Source: CAD feature listing. Evaluate the final solid. Frame: model axes, mm. A direction names the side the tool comes from. Coordinates: 2 decimals unless noted, no trailing zeros. Write each loop counter-clockwise with the first axis right and the second up, starting at its lowest first coordinate (ties: lowest second). Pieces come first, ordered by that corner, then holes. Notation, with made-up numbers: (23.5, 73) - (44.5, 73) arc R22 ccw to (44.5, 98) - close; hole circle Ø3 at (-10, 60.5). An arc over 180 degrees is marked (long way). One line per question, with ' | ' between items.
from build123d import *

# Parameters (mm, degrees)
SKETCH1_W            = 35
SKETCH1_H            = 15
BASE_FLANGE1_DEPTH   = 2
EDGE_FLANGE1_START   = -17.5
EDGE_FLANGE1_DEPTH   = 35
EDGE_FLANGE1_2_DEPTH = 35
EDGE_FLANGE2_START   = -17.5
EDGE_FLANGE2_DEPTH   = 35
EDGE_FLANGE2_2_DEPTH = 35
SKETCH8_W            = 25
SKETCH8_H            = 56.677305051
CUT_EXTRUDE1_DEPTH   = 10
BOSS_EXTRUDE1_DEPTH  = 2
BOSS_EXTRUDE2_DEPTH  = 2
M3_CLEARANCE_HOLE1_D = 3.6
M3_CLEARANCE_HOLE2_D = 3.6
M3_CLEARANCE_HOLE3_D = 3.6
M3_CLEARANCE_HOLE4_D = 3.6


# Read off the part's stored shape, not the designer's step: Edge-Flange1, Edge-Flange2
# Sheet-metal steps are written as plain solids
with BuildPart() as part:
    # Sketch1 → Base-Flange1 (new body)
    with BuildSketch(Plane.XY):
        Rectangle(SKETCH1_W, SKETCH1_H)
    extrude(amount=-BASE_FLANGE1_DEPTH)

    # Edge-Flange1 outline → Edge-Flange1 (cut)
    with BuildSketch(Plane.YZ.offset(EDGE_FLANGE1_START)):
        with BuildLine():
            ThreePointArc((-2.964101615, -2), (-3.999377795, -1.863703305), (-4.964101615, -1.464101615))
            Line((-4.964101615, -1.464101615), (-7.5, 0))
            Line((-7.5, 0), (-7.5, -2))
            Line((-7.5, -2), (-2.964101615, -2))
        make_face()
    extrude(amount=EDGE_FLANGE1_DEPTH, mode=Mode.SUBTRACT)

    # Edge-Flange1 2 outline → Edge-Flange1 2 (add)
    with BuildSketch(Plane.YZ.offset(EDGE_FLANGE1_START)):
        with BuildLine():
            Line((-65.708341645, 33.606601718), (-7.5, 0))
            Line((-7.5, 0), (-2.964101615, 0))
            ThreePointArc((-2.964101615, 0), (-3.481739705, 0.068148347), (-3.964101615, 0.267949192))
            Line((-3.964101615, 0.267949192), (-64.708341645, 35.338652525))
            Line((-64.708341645, 35.338652525), (-65.708341645, 33.606601718))
        make_face()
    extrude(amount=EDGE_FLANGE1_2_DEPTH)

    # Edge-Flange2 outline → Edge-Flange2 (cut)
    with BuildSketch(Plane.YZ.offset(EDGE_FLANGE2_START)):
        with BuildLine():
            ThreePointArc((-62.708341645, 31.87455091), (-64.17244326, 33.338652525), (-64.708341645, 35.338652525))
            Line((-64.708341645, 35.338652525), (-65.708341645, 33.606601718))
            Line((-65.708341645, 33.606601718), (-62.708341645, 31.87455091))
        make_face()
    extrude(amount=EDGE_FLANGE2_DEPTH, mode=Mode.SUBTRACT)

    # Edge-Flange2 2 outline → Edge-Flange2 2 (add)
    with BuildSketch(Plane.YZ.offset(EDGE_FLANGE2_START)):
        with BuildLine():
            Line((-64.708341645, 48.029251449), (-64.708341645, 35.338652525))
            Line((-64.708341645, 35.338652525), (-61.708341645, 33.606601718))
            ThreePointArc((-61.708341645, 33.606601718), (-62.440392453, 34.338652525), (-62.708341645, 35.338652525))
            Line((-62.708341645, 35.338652525), (-62.708341645, 48.029251449))
            Line((-62.708341645, 48.029251449), (-64.708341645, 48.029251449))
        make_face()
    extrude(amount=EDGE_FLANGE2_2_DEPTH)

    # Sketch8 → Cut-Extrude1 (cut)
    with BuildSketch(Plane(origin=(0, -0.875, -1.515544457), x_dir=(1, 0, 0), z_dir=(0, 0.499999999999995, 0.8660254037844416))):
        with Locations((0, -36.905639824)):
            Rectangle(SKETCH8_W, SKETCH8_H)
    extrude(amount=-CUT_EXTRUDE1_DEPTH, mode=Mode.SUBTRACT)

    # Sketch9 → Boss-Extrude1 (add)
    with BuildSketch(Plane(origin=(0, -0.875, -1.515544457), x_dir=(1, 0, 0), z_dir=(0, 0.499999999999995, 0.8660254037844416))):
        Polygon((8.83956854, -68.632858088), (7.246458748, -62.687291403), (15.857586038, -60.3799468), (15.081128903, -57.482169321), (6.470001613, -59.789513924), (1.919269462, -42.805950327), (15.365688048, -39.202993325), (14.946719777, -36.202993325), (1.14120391, -39.902170153), (-2.665166674, -25.696601742), (16.123001013, -20.662327383), (15.50761088, -17.662327383), (-3.456389996, -22.743716103), (-8.33426209, -4.539249615), (-11.232039569, -5.31570675), (-8.495960417, -15.52689316), (-17.05592393, -17.82052847), (-16.279466794, -20.718305949), (-7.708625485, -18.465267128), (-3.822054178, -32.970148713), (-15.793222539, -36.177813607), (-15.040127716, -39.177813607), (-3.021606391, -35.957460524), (1.177204702, -51.627636855), (-15.406874361, -56.071327447), (-14.947395895, -59.071327447), (1.957983923, -54.541544577), (5.941791061, -69.409315224), align=None)
    extrude(amount=-BOSS_EXTRUDE1_DEPTH)

    # Sketch10 → Boss-Extrude2 (add)
    with BuildSketch(Plane(origin=(0, -0.875, -1.515544457), x_dir=(1, 0, 0), z_dir=(0, 0.499999999999995, 0.8660254037844416))):
        Polygon((-3.456389996, -22.743716103), (12.5, -8.566987298), (10.507436864, -6.324289782), (-5.448953132, -20.501018587), align=None)
        Polygon((-2.665166674, -25.696601742), (12.5, -36.858589914), (14.278322137, -34.442483464), (-0.886844536, -23.280495293), align=None)
        Polygon((-3.822054178, -32.970148713), (-12.5, -19.724787915), (-15.00938766, -21.368860167), (-6.331441838, -34.614220965), align=None)
        Polygon((-12.5, -55.29243281), (-3.021606391, -35.957460524), (-5.715342898, -34.636936526), (-15.193736507, -53.971908812), align=None)
        Polygon((6.470001613, -59.789513924), (12.5, -39.970852124), (15.37009296, -40.844102603), (9.340094573, -60.662764404), align=None)
        Polygon((-12.5, -58.415549694), (4.825776546, -65.244292349), (3.725723751, -68.035328689), (-13.600052794, -61.206586033), align=None)
    extrude(amount=-BOSS_EXTRUDE2_DEPTH)

    # M3 Clearance Hole1 (through all)
    with Locations(Plane(origin=(-15.830402425, -63.569767603, -87), x_dir=(-1, 0, 0), z_dir=(0, 0, -1))):
        with Locations((-25.330402425, 65.569767603), (-6.330402425, 65.739876607)):
            Hole(M3_CLEARANCE_HOLE1_D / 2)

    # M3 Clearance Hole2 (through all)
    with Locations(Plane(origin=(15.830402425, -63.569767603, 0), x_dir=(1, 0, 0), z_dir=(0, 0, 1))):
        with Locations((-25.330402425, 65.569767603), (-6.330402425, 65.739876607)):
            Hole(M3_CLEARANCE_HOLE2_D / 2)

    # M3 Clearance Hole3 (through all)
    with Locations(Plane(origin=(15.830402425, -62.708341645, 22.375161803), x_dir=(-1, 0, 0), z_dir=(0, 1, 0))):
        with Locations((25.330402425, 19.654089646), (6.330402425, 19.654089646)):
            Hole(M3_CLEARANCE_HOLE3_D / 2)

    # M3 Clearance Hole4 (through all)
    with Locations(Plane(origin=(-15.830402425, -62.708341645, -109.375161803), x_dir=(1, 0, 0), z_dir=(0, 1, 0))):
        with Locations((25.330402425, -151.404413252), (6.330402425, -151.404413252)):
            Hole(M3_CLEARANCE_HOLE4_D / 2)


solid = part.part
Item 1: Pin query (flat end, axial travel): pin 1 Ø11.5 at (x, y) = (-1.5, 3.5) entering from +Z; pin 2 Ø1 at (x, y) = (6, -7) entering from -Z; pin 3 Ø14 at (x, z) = (-6, 43.5) entering from +Y. Return the tip coordinate at first contact, or that it passes through.
Check sheet entries:
pin 1: z = 0 | pin 2: z = -0.58 | pin 3: y = -62.71
Item 2: Ray query, line 1 along Y through (x, z) = (-7, 44.5); line 2 along Z through (x, y) = (9.5, -63.45); line 3 along Z through (x, y) = (9, -64). Return the intervals inside material, ascending. Write a range as [from, to].
Check sheet entries:
line 1: [-64.71, -62.71] | line 2: [32.43, 40.23], [43.83, 48.03] | line 3: [33.07, 40.3], [43.76, 48.03]
Item 3: Mould query, pull axis X, two halves, no side actions, for faces 3 (the face through (-17.5, -37, 18)), 4 (the face through (0, 2, 0)), 5 (the face through (-0.735, -29.859, 14.08)). Classes: pulls with the +X half, pulls with the -X half, needs draft (parallel to the pull), parting line crosses it, or undercut.
Check sheet entries:
face 3: pulls with the -X half | face 4: needs draft | face 5: undercut
Item 4: Cut plane A-A on x = 0. State how many separate pieces and enclosed holes the cut face has, and give its area (3 significant figures).
Check sheet entries:
separate pieces: 6 | enclosed holes: 0 | area: 129 mm²
Item 5: Cut plane C-C on z = 2. Return loops of the section in (x, y).
Check sheet entries:
outline: (-17.5, -10.96) - (-12.5, -10.96) - (-12.5, -8.74) - (-10.36, -8.74) - (-9.84, -10.96) - (-6.74, -10.96) - (-7.26, -8.74) - (7.98, -8.74) - (5.81, -10.96) - (10.33, -10.96) - (12.5, -8.74) - (12.5, -10.96) - (17.5, -10.96) - (17.5, -6.96) - (-17.5, -6.96) - close
Item 6: Access query for faces 1 (the face through (9.5, 0.2, -1)), 2 (the face through (12.5, -56, 29)). Directions: +Z, -Z, +X, -X, +Y, -Y. A direction counts if a zero-diameter tool reaches every point of the face in a straight line with its end or side. Return the directions, or none.
Check sheet entries:
face 1: +Z, -Z | face 2: none
Item 7: Cut plane B-B on y = -27.5. Return loops of the section in (x, z), and give its area (3 significant figures).
Check sheet entries:
outline: (-17.5, 11.55) - (-12.5, 11.55) - (-12.5, 13.86) - (-17.5, 13.86) - close; (-9.62, 11.55) - (-6.04, 11.55) - (-5.28, 13.86) - (-8.87, 13.86) - close; (-4.73, 11.55) - (-1.62, 11.55) - (-1.31, 13.86) - (-4.42, 13.86) - close; (2.62, 11.55) - (7.68, 11.55) - (9.25, 13.86) - (4.19, 13.86) - close; (12.5, 11.55) - (17.5, 11.55) - (17.5, 13.86) - (12.5, 13.86) - close | area: 50.2 mm²
